from build123d import *

# Parameters (mm, degrees)
SKETCH1_W             = 170
SKETCH1_H             = 97
BOSS_EXTRUDE1_DEPTH   = 30
FILLET1_R             = 5
SKETCH2_W             = 70.1
SKETCH2_H             = 55.1
CUT_EXTRUDE3_DEPTH    = 103.358438831
F_8_0MM_DOWEL_HOLE1_D = 8
M8_CLEARANCE_HOLE1_D  = 8.4


with BuildPart() as part:
    # Sketch1 → Boss-Extrude1 (new body)
    with BuildSketch(Plane(origin=(0, 0, 0), x_dir=(1, 0, 0), z_dir=(0, 1, 0))):
        Rectangle(SKETCH1_W, SKETCH1_H)
    extrude(amount=-BOSS_EXTRUDE1_DEPTH)

    # Fillet1
    fillet1_edges = [part.edges().sort_by_distance(p)[0] for p in [
        (85, -15, 48.5),
        (-85, -15, 48.5),
        (-85, -15, -48.5),
        (85, -15, -48.5),
    ]]
    fillet(fillet1_edges, radius=FILLET1_R)

    # Sketch2 → Cut-Extrude3 (cut, through all)
    with BuildSketch(Plane(origin=(0, -30, 0), x_dir=(1, 0, 0), z_dir=(0, 1, 0))):
        Rectangle(SKETCH2_W, SKETCH2_H)
    extrude(amount=CUT_EXTRUDE3_DEPTH, mode=Mode.SUBTRACT)

    # Ø8.0mm Dowel Hole1 (through all)
    with Locations(Plane(origin=(0, 0, 0), x_dir=(1, 0, 0), z_dir=(0, 1, 0))):
        with Locations((-75, 0), (75, 0)):
            Hole(F_8_0MM_DOWEL_HOLE1_D / 2)

    # M8 Clearance Hole1 (through all)
    with Locations(Plane(origin=(0, 0, 0), x_dir=(1, 0, 0), z_dir=(0, 1, 0))):
        with Locations((-75, 38.5), (-75, -38.5), (75, -38.5), (75, 38.5)):
            Hole(M8_CLEARANCE_HOLE1_D / 2)


solid = part.part
Source: CAD feature listing. Evaluate the final solid. Frame: model axes, mm. A direction names the side the tool comes from. Give positions to 0.01 mm unless a question says otherwise; leave off trailing zeros. Order: outer loops, then holes, each group sorted by start corner. A loop starts at its lowest first (then second) coordinate and runs counter-clockwise, first axis right, second up. Notation, with made-up numbers: (59, 14) -> (116, 14) arc R22 ccw to (116, 53) -> close; hole circle Ø11 at (58, -18). An arc over 180 degrees is marked (long way). Write item = value, one per line.
Item 1: Section query B-B (x = -18.5). Output: boundary loops of the cut face in (y, z), then the cut area to 3 significant figures.
Check result:
outline = (-30, -48.5) -> (0, -48.5) -> (0, -27.55) -> (-30, -27.55) -> close; (-30, 27.55) -> (0, 27.55) -> (0, 48.5) -> (-30, 48.5) -> close
area = 1,260 mm²
Item 2: Contact query for a flat-ended pin moving along its axis: pin 1 (5 mm diameter, centred on x = -75, z = 0, fed in from -Y). Output: stop coordinate, or through.
Check result:
pin_1 = through
Item 3: Ray query, probe 1 along Z at (x, y) = (-75, -6.25); probe 2 along X at (y, z) = (-1.25, 6); probe 3 along Z at (x, y) = (19, -18.25). Return the intervals inside material, ascending.
Check result:
probe_1 = -48.5 to -42.7, -34.3 to -4, 4 to 34.3, 42.7 to 48.5
probe_2 = -85 to -35.05, 35.05 to 85
probe_3 = -48.5 to -27.55, 27.55 to 48.5
Item 4: Section query D-D (z = 0). Output: boundary loops of the cut face in (x, y), then the cut area to 3 significant figures.
Check result:
outline = (-85, -30) -> (-79, -30) -> (-79, 0) -> (-85, 0) -> close; (-71, -30) -> (-35.05, -30) -> (-35.05, 0) -> (-71, 0) -> close; (35.05, -30) -> (71, -30) -> (71, 0) -> (35.05, 0) -> close; (79, -30) -> (85, -30) -> (85, 0) -> (79, 0) -> close
area = 2,520 mm²
Item 5: Section query C-C (y = -2.5). Output: boundary loops of the cut face in (x, z), then the cut area to 3 significant figures.
Check result:
outline = (-85, -43.5) arc R5 ccw to (-80, -48.5) -> (80, -48.5) arc R5 ccw to (85, -43.5) -> (85, 43.5) arc R5 ccw to (80, 48.5) -> (-80, 48.5) arc R5 ccw to (-85, 43.5) -> close; hole circle Ø8.4 at (-75, -38.5); hole circle Ø8.4 at (-75, 38.5); hole circle Ø8 at (-75, 0); hole (-35.05, -27.55) -> (35.05, -27.55) -> (35.05, 27.55) -> (-35.05, 27.55) -> close; hole circle Ø8.4 at (75, -38.5); hole circle Ø8.4 at (75, 38.5); hole circle Ø8 at (75, 0)
area = 12,300 mm²
Item 6: Mould query, pull axis Z, two halves, no side actions, for faces 3 (the face through (78.096, -15.21, 35.661)), 4 (the face through (-1, -15, -48.5)), 5 (the face through (79.196, -15.21, -38.685)), 6 (the face through (83.5, -15.21, 47.07)). Classes: +Z half, -Z half, draft (parallel to the pull), parting line (faces both ways), or undercut.
Check result:
face_3 = undercut
face_4 = -Z half
face_5 = undercut
face_6 = +Z half
Item 7: Section query A-A (z = -11.5). Output: boundary loops of the cut face in (x, y).
Check result:
outline = (-85, -30) -> (-35.05, -30) -> (-35.05, 0) -> (-85, 0) -> close; (35.05, -30) -> (85, -30) -> (85, 0) -> (35.05, 0) -> close
Item 8: Set-up query: faces 1 (the face through (0, -15, -27.55)), 2 (the face through (-1, 0, -33)). Return all of +Z, -Z, +X, -X, +Y, -Y with unobstructed straight access to the full face (end or side cutting, diameter ignored); none if empty.
Check result:
face_1 = +Y, -Y
face_2 = +Z, -Z, +X, -X, +Y
